```python
from build123d import *

# Parameters (mm, degrees)
F0_W      = 16
F0_H      = 16
F1_DEPTH  = 8
F2_R      = 1.75
F3_DEPTH  = 1
F4_R      = 1.75
F5_DEPTH  = 1
F6_R      = 1.75
F7_DEPTH  = 1
F8_R      = 1
F9_R      = 1.75
F10_DEPTH = 1
F11_R     = 1.75
F12_DEPTH = 1
F13_R     = 1.75
F14_DEPTH = 1


with BuildPart() as f1:
    # F0 (on Front) → F1 (new body, symmetric)
    with BuildSketch(Plane.XZ):
        Rectangle(F0_W, F0_H)
    extrude(amount=F1_DEPTH, both=True)

    # F2 (on face) → F3 (cut)
    with BuildSketch(Plane.XZ.offset(8)):
        with Locations((5, 5)):
            Circle(F2_R)
        with Locations((-5, -5)):
            Circle(F2_R)
    extrude(amount=-F3_DEPTH, mode=Mode.SUBTRACT)

    # F4 (on face) → F5 (cut)
    with BuildSketch(Plane.YZ.offset(8)):
        with Locations((-5, 5)):
            Circle(F4_R)
        with Locations((-5, 0)):
            Circle(F4_R)
        with Locations((-5, -5)):
            Circle(F4_R)
        with Locations((5, 5)):
            Circle(F4_R)
        with Locations((5, 0)):
            Circle(F4_R)
        with Locations((5, -5)):
            Circle(F4_R)
    extrude(amount=-F5_DEPTH, mode=Mode.SUBTRACT)

    # F6 (on face) → F7 (cut)
    with BuildSketch(Plane.XY.offset(8)):
        with Locations((-5, 5)):
            Circle(F6_R)
        with Locations((5, -5)):
            Circle(F6_R)
        Circle(F6_R)
    extrude(amount=-F7_DEPTH, mode=Mode.SUBTRACT)

    # F8
    f8_edges = [f1.edges().sort_by_distance(p)[0] for p in [
        (0, -8, 8),
        (8, 0, 8),
        (8, -8, 0),
        (8, 8, 0),
        (8, 0, -8),
        (0, 8, 8),
        (-8, 0, 8),
        (-8, 8, 0),
        (0, 8, -8),
        (-8, 0, -8),
        (0, -8, -8),
        (-8, -8, 0),
    ]]
    fillet(f8_edges, radius=F8_R)

    # F9 (on face) → F10 (cut)
    with BuildSketch(Plane(origin=(-8, 0, 0), x_dir=(0, -1, 0), z_dir=(-1, 0, 0))):
        Circle(F9_R)
    extrude(amount=-F10_DEPTH, mode=Mode.SUBTRACT)

    # F11 (on face) → F12 (cut)
    with BuildSketch(Plane(origin=(0, 8, 0), x_dir=(-1, 0, 0), z_dir=(0, 1, 0))):
        with Locations((-5, 5)):
            Circle(F11_R)
        with Locations((-5, -5)):
            Circle(F11_R)
        with Locations((5, 5)):
            Circle(F11_R)
        with Locations((5, -5)):
            Circle(F11_R)
        Circle(F11_R)
    extrude(amount=-F12_DEPTH, mode=Mode.SUBTRACT)

    # F13 (on face) → F14 (cut)
    with BuildSketch(Plane(origin=(0, 0, -8), x_dir=(1, 0, 0), z_dir=(0, 0, -1))):
        with Locations((-5, 5)):
            Circle(F13_R)
        with Locations((5, 5)):
            Circle(F13_R)
        with Locations((5, -5)):
            Circle(F13_R)
        with Locations((-5, -5)):
            Circle(F13_R)
    extrude(amount=-F14_DEPTH, mode=Mode.SUBTRACT)


solid = f1.part
```
Input: part model. Units: mm. Frame: model coordinates. A direction names the side the tool comes from. Coordinates: 2 decimals unless noted, no trailing zeros. Loops run counter-clockwise (first coordinate to the right, second up) from the corner with the lowest first, then second, coordinate; pieces in that order, holes last.
Q1. Section D-D, the plane z = 7.25. Return the cut outline in (x, y).
Results are:
outline: (-7.97, -7) arc R0.97 ccw to (-7, -7.97) - (7, -7.97) arc R0.97 ccw to (7.97, -7) - (7.97, 7) arc R0.97 ccw to (7, 7.97) - (-7, 7.97) arc R0.97 ccw to (-7.97, 7) - close; hole circle Ø3.5 at (-5, 5); hole circle Ø3.5 at (0, 0); hole circle Ø3.5 at (5, -5)
Q2. Set-up query: faces 4 (the cylindrical face through (-7.507, -1.617, -0.67)), 5 (the flat face through (7, 5, -5)), 6 (the cylindrical face through (3.61, -3.94, -7.51)). Return all of +Z, -Z, +X, -X, +Y, -Y with unobstructed straight access to the full face (end or side cutting, diameter ignored); none if empty.
Results are:
face 4: -X
face 5: +X
face 6: -Z
Q3. Contact query for flat-ended pins moving along their axis: pin 1 (3 mm diameter, centred on x = -5, y = -5, fed in from -Z); pin 2 (3 mm diameter, centred on x = -5, z = -5, fed in from -Y); pin 3 (4 mm diameter, centred on x = 5, z = 5, fed in from +Y); pin 4 (3 mm diameter, centred on x = -5, z = 5, fed in from +Y). Output: stop coordinate, or through.
Results are:
pin 1: stops at z = -7
pin 2: stops at y = -7
pin 3: stops at y = 8
pin 4: stops at y = 7
Q4. Line query: line 1 along Z through (x, y) = (7.85, 5); line 2 along Z through (x, y) = (7.25, -5); line 3 along Y through (x, z) = (-5, -7.55). Output: solid intervals per line, ascending.
Results are:
line 1: z = -7.53 to -6.75, -3.25 to -1.75, 1.75 to 3.25, 6.75 to 7.53
line 2: z = -7.97 to -6.75, -3.25 to -1.75, 1.75 to 3.25, 6.75 to 7.97
line 3: y = -7.84 to -6.75, -3.25 to 3.25, 6.75 to 7.84
Q5. Mould query, pull axis X, two halves, no side actions, for faces 1 (the cylindrical face through (-7.715, 7.699, 0.098)), 2 (the cylindrical face through (7.51, -5.38, -6.71)), 3 (the flat face through (5, -7, 5)). Classes: +X half, -X half, draft (parallel to the pull), parting line (faces both ways), or undercut.
Results are:
face 1: -X half
face 2: draft
face 3: undercut
Q6. Section C-C, the plane x = 0. Return the cut outline in (y, z).
Results are:
outline: (-8, -7) arc R1 ccw to (-7, -8) - (7, -8) arc R1 ccw to (8, -7) - (8, -1.75) - (7, -1.75) - (7, 1.75) - (8, 1.75) - (8, 7) arc R1 ccw to (7, 8) - (1.75, 8) - (1.75, 7) - (-1.75, 7) - (-1.75, 8) - (-7, 8) arc R1 ccw to (-8, 7) - close
Q7. Section A-A, the plane z = 0. Return the cut outline in (x, y), and give its area (3 significant figures).
Results are:
outline: (-8, -7) arc R1 ccw to (-7, -8) - (7, -8) arc R1 ccw to (8, -7) - (8, -6.75) - (7, -6.75) - (7, -3.25) - (8, -3.25) - (8, 3.25) - (7, 3.25) - (7, 6.75) - (8, 6.75) - (8, 7) arc R1 ccw to (7, 8) - (1.75, 8) - (1.75, 7) - (-1.75, 7) - (-1.75, 8) - (-7, 8) arc R1 ccw to (-8, 7) - (-8, 1.75) - (-7, 1.75) - (-7, -1.75) - (-8, -1.75) - close
area: 241 mm2
Q8. Section B-B, the plane y = 0. Return the cut outline in (x, z), and give its area (3 significant figures).
Results are:
outline: (-8, -7) arc R1 ccw to (-7, -8) - (7, -8) arc R1 ccw to (8, -7) - (8, 7) arc R1 ccw to (7, 8) - (1.75, 8) - (1.75, 7) - (-1.75, 7) - (-1.75, 8) - (-7, 8) arc R1 ccw to (-8, 7) - (-8, 1.75) - (-7, 1.75) - (-7, -1.75) - (-8, -1.75) - close
area: 248 mm2
